Solid Edge part; units mm, degrees
sketch "Sketch1" plane through (0, 0, 0) normal (0, 0, 1) x (1, 0, 0)
  circle A0 centre (0, 0) radius 101.5
extrude "Protrusion1" add sketch "Sketch1" along normal blind 19
sketch "Sketch2" plane through (0, 0, 19) normal (0, 0, 1) x (1, 0, 0)
  circle A0 centre (0, 86) radius 8
extrude "ExtrudedCutout_1" cut sketch "Sketch2" against normal blind 93.7971
pattern_circular "Pattern1" count 6 over 360 about axis through (0, 0, 19) along (0, 0, -1) of "ExtrudedCutout_1"
sketch "Sketch3" plane through (0, 0, 19) normal (0, 0, 1) x (1, 0, 0)
  circle A0 centre (0, 0) radius 32
extrude "ExtrudedProtrusion_2" add sketch "Sketch3" along normal blind 51
sketch "Sketch4" plane through (0, 0, 70) normal (0, 0, 1) x (1, 0, 0)
  circle A0 centre (0, 0) radius 16
extrude "ExtrudedCutout_2" cut sketch "Sketch4" against normal blind 138.4469
sketch "Sketch5" plane through (0, 0, 0) normal (0, -1, 0) x (1, 0, 0)
  line L0 (-32, 70) -> (-123.1874, 37.1288)
  line L1 (0, 0) -> (-117.5, 0)
  line L2 (0, 19) -> (0, 0)
  line L3 (-16, 19) -> (0, 19)
  line L4 (-16, 70) -> (-16, 19)
  line L5 (-32, 70) -> (-16, 70)
  arc A0 (-117.5, 0) -> (-123.1874, 37.1288) centre (-117.5, 19) cw
  circle A1 centre (-117.5, 19) radius 6.5
extrude "ExtrudedProtrusion_5" add sketch "Sketch5" along normal mid plane 16
pattern_circular "Pattern3" count 3 over 360 about axis through (0, 0, 19) along (0, 0, -1) of "ExtrudedProtrusion_5"
sketch "Sketch6" plane through (0, 0, 70) normal (0, 0, 1) x (1, 0, 0)
  circle A0 centre (0, 0) radius 16
extrude "ExtrudedCutout_3" cut sketch "Sketch6" along normal mid plane 22491.7976
Can you work these out from the model? Positions are in its coordinate system, mm. A direction names the side the tool comes from. Give positions to 0.01 mm unless a question says otherwise; leave off trailing zeros. Order: outer loops, then holes, each group sorted by start corner. A loop starts at its lowest first (then second) coordinate and runs counter-clockwise, first axis right, second up. Notation, with made-up numbers: M 44.25,-33.75 L 98.25,-33.75 A17 cw 98.25,-10.75 Z; hole C -31.5,76.5 d8. An arc over 180 degrees is marked long. Use a Markdown table: item, result. Add a question column.
Item 1: Suppose I cut it at B-B (x = 0). List the corners of the cut face in (y, z) for me.
Item 2: We'd pull the mould along Y, two halves only. Please class faces 6 (the flat face through (-10, 25, 0)), 7 (the cylindrical face through (-68.13, 47.87, 9.63)), 8 (the flat face through (38.381, -66.701, 53.794)): +Y half, -Y half, draft (parallel to the pull), parting line (faces both ways), or undercut.
Item 3: For faces 1 (the flat face through (61, 1, 19)), 2 (the flat face through (-71, -8, 35)), 3 (the flat face through (-71, 8, 35)), 4 (the cylindrical face through (-49.554, -88.581, 9.367)), 5 (the cylindrical face through (-80.37, -37.59, 9.63)), which set-ups out of +Z, -Z, +X, -X, +Y, -Y let a thin tool reach every point of the face, with its end or its side?
Item 4: Will these pins go through, and if not, where does the flat tip stop? pin 1 (12 mm diameter, centred on x = 55, z = 59.5, fed in from -Y); pin 2 (10 mm diameter, centred on x = 9, z = 29, fed in from -Y); pin 3 (2 mm diameter, centred on x = 63.5, z = 23.5, fed in from +Y); pin 4 (4 mm diameter, centred on x = -26, z = 33, fed in from +Y).
Item 5: Suppose I cut it at A-A (z = 16). Count the separate pieces of the cut face and the enclosed holes in it, then the cut area to 3 significant figures.
Item 6: Suppose I cut it at C-C (y = -43). List the corners of the cut face in (x, z) for me, then the cut area to 3 significant figures.
Item 7: If I drill on L1, parallel to Y at x = 0, z = 15; L2, parallel to Y at x = 5, z = 5 (3 decimals); L3, parallel to Z at x = -54.5, y = 57.5, over which ranges is the centre line in solid material (lowest first)? Write a range as [from, to].
Item 8: Suppose I cut it at D-D (z = 30.5). List the corners of the cut face in (x, y) for me.
Answer sheet:
| question | item | result |
|---|---|---|
| 1 | outline | M -101.5,0 L -94,0 L -94,19 L -101.5,19 Z; M -78,0 L -16,0 L -16,70 L -32,70 L -32,19 L -78,19 Z; M 16,0 L 78,0 L 78,19 L 32,19 L 32,70 L 16,70 Z; M 94,0 L 101.5,0 L 101.5,19 L 94,19 Z |
| 2 | face 6 | draft |
| 2 | face 7 | undercut |
| 2 | face 8 | -Y half |
| 3 | face 1 | +Z, +X |
| 3 | face 2 | +Z, -X, -Y |
| 3 | face 3 | +Z, -X, +Y |
| 3 | face 4 | +Z, -Z, -Y |
| 3 | face 5 | +Z, -Z |
| 4 | pin 1 | passes through |
| 4 | pin 2 | stops at y = -40.25 |
| 4 | pin 3 | stops at y = 120.97 |
| 4 | pin 4 | stops at y = 21.17 |
| 5 | separate pieces | 4 |
| 5 | enclosed holes | 7 |
| 5 | area | 31,500 mm² |
| 6 | outline | M -91.94,0 L -82.48,0 L -82.48,19 L -91.94,19 Z; M -66.48,0 L 66.48,0 L 66.48,19 L 34.06,19 L 34.06,61.97 L 15.59,65.3 L 15.59,19 L -66.48,19 Z; M 82.48,0 L 91.94,0 L 91.94,19 L 82.48,19 Z |
| 6 | area | 3,710 mm² |
| 7 | L1 | y = [-101.5, -94], [-78, -16], [16, 78], [94, 101.5] |
| 7 | L2 | y = [-101.377, -92.245], [-79.755, -15.199], [15.199, 79.755], [92.245, 101.377] |
| 7 | L3 | z = [0, 19] |
| 8 | outline | M -132.62,-8 L -30.98,-8 A32 ccw 8.56,-30.83 L 59.38,-118.86 L 73.24,-110.86 L 22.42,-22.83 A32 ccw 22.42,22.83 L 73.24,110.86 L 59.38,118.86 L 8.56,30.83 A32 ccw -30.98,8 L -132.62,8 Z; hole C 0,0 d32 |
